Can you work these out from the model? Positions are in its coordinate system, mm. Coordinates: 2 decimals unless noted, no trailing zeros. Order: outer loops, then holes, each group sorted by start corner. A loop starts at its lowest first (then second) coordinate and runs counter-clockwise, first axis right, second up. Notation, with made-up numbers: (26, 39) -> (85, 39) arc R19 cw to (85, 71) -> close; hole circle Ø4 at (60.5, 72.25). An arc over 180 degrees is marked (long way). Answer as a JSON object with one key per item and string values. Group by question number.
(1) If we mould it in two halves opening along X, with no side actions, what happens to faces 1 (the cylindrical face through (30.228, 5.76, -0.522)), 2 (the flat face through (-4, 0, -18)), 3 (the flat face through (2, 0, 2)), 4 (the cylindrical face through (-0.522, 5.76, -30.228))? For each: pulls with the +X half, pulls with the -X half, needs draft (parallel to the pull), parting line crosses it, or undercut.
(2) For pin 1 (3 mm diameter, centred on x = 14, y = -0.5, fed in from +Z); pin 2 (5 mm diameter, centred on y = 0, z = -17, fed in from -X); pin 3 (1.5 mm diameter, centred on y = -0.5, z = 14.5, fed in from +X); pin 4 (12 mm diameter, centred on x = 19.5, z = 12, fed in from -Y), each with a flat end and sliding along its axis, tell me the tip position at first contact or that it passes through.
(3) I want a section at A-A, the plane y = 1.75. List the corners of the cut face in (x, z) for me.
(4) I want a section at C-C, the plane x = -14. List the corners of the cut face in (y, z) for me, plus the area to 3 significant figures.
(5) I need wall thicknesses on line 1 (X direction, y = 10, z = -3); line 2 (X direction, y = 5, z = -1); line 3 (Z direction, x = -16, y = -1). Which ranges of each line are inside material? Lowest first, please.
(6) I want a section at B-B, the plane y = 5.75. List the corners of the cut face in (x, z) for me.
from build123d import *

# Parameters (mm, degrees)
BOSS_EXTRU_1_DEPTH           = 3
BOSS_EXTRU_1_DEPTH_BACK      = 3
BOSS_EXTRU_2_START           = -6
ESQUISSE2_R                  = 4.01172956
BOSS_EXTRU_2_DEPTH           = 14.5
R_P_TITION_CIRCULAIRE1_COUNT = 4
ESQUISSE3_R                  = 1.05
ENL_V_MAT_EXTRU_1_DEPTH      = 43.796548364
ENL_V_MAT_EXTRU_1_DEPTH_BACK = 43.796548364
ENL_V_MAT_EXTRU_2_DEPTH      = 12.5
ENL_V_MAT_EXTRU_2_DEPTH_BACK = 4.0000001


with BuildPart() as part:
    # Esquisse1 → Boss.-Extru.1 (new body, two sides)
    with BuildSketch(Plane(origin=(0, 0, 0), x_dir=(1, 0, 0), z_dir=(0, 1, 0))) as boss_extru_1_sk:
        with BuildLine():
            Line((4, -25.943448113), (4, -9.16515139))
            ThreePointArc((4, -9.16515139), (7.071067812, -7.071067812), (9.16515139, -4))
            Line((9.16515139, -4), (25.943448113, -4))
            ThreePointArc((25.943448113, -4), (26.25, 0), (25.943448113, 4))
            Line((25.943448113, 4), (9.16515139, 4))
            ThreePointArc((9.16515139, 4), (7.071067812, 7.071067812), (4, 9.16515139))
            Line((4, 9.16515139), (4, 25.943448113))
            ThreePointArc((4, 25.943448113), (0, 26.25), (-4, 25.943448113))
            Line((-4, 25.943448113), (-4, 9.16515139))
            ThreePointArc((-4, 9.16515139), (-7.071067812, 7.071067812), (-9.16515139, 4))
            Line((-9.16515139, 4), (-25.943448113, 4))
            ThreePointArc((-25.943448113, 4), (-26.25, 0), (-25.943448113, -4))
            Line((-25.943448113, -4), (-9.16515139, -4))
            ThreePointArc((-9.16515139, -4), (-7.071067812, -7.071067812), (-4, -9.16515139))
            Line((-4, -9.16515139), (-4, -25.943448113))
            ThreePointArc((-4, -25.943448113), (0, -26.25), (4, -25.943448113))
        make_face()
    extrude(amount=BOSS_EXTRU_1_DEPTH)
    extrude(boss_extru_1_sk.sketch, amount=-BOSS_EXTRU_1_DEPTH_BACK)

    # Esquisse2 → Boss.-Extru.2 (add)
    with BuildSketch(Plane(origin=(0, 3, 0), x_dir=(1, 0, 0), z_dir=(0, 1, 0)).offset(BOSS_EXTRU_2_START)):
        with Locations((0, 26.25)):
            Circle(ESQUISSE2_R)
    boss_extru_2 = extrude(amount=BOSS_EXTRU_2_DEPTH)

    # Répétition circulaire1: Boss.-Extru.2 ×4 about axis
    r_p_tition_circulaire1_axis = Axis((0, 0, 0), (0, 1, 0))
    for i in range(1, R_P_TITION_CIRCULAIRE1_COUNT):
        add(boss_extru_2.rotate(r_p_tition_circulaire1_axis, i * 360 / R_P_TITION_CIRCULAIRE1_COUNT))

    # Esquisse3 → Enlèv. mat.-Extru.1 (cut, two sides)
    with BuildSketch(Plane(origin=(0, 0, 0), x_dir=(-0.707106781, 0, -0.707106781), z_dir=(0.707106781, 0, -0.707106781))) as enl_v_mat_extru_1_sk:
        Circle(ESQUISSE3_R)
    extrude(amount=ENL_V_MAT_EXTRU_1_DEPTH, mode=Mode.SUBTRACT)
    extrude(enl_v_mat_extru_1_sk.sketch, amount=-ENL_V_MAT_EXTRU_1_DEPTH_BACK, mode=Mode.SUBTRACT)

    # Esquisse4 → Enlèv. mat.-Extru.2 (cut, two sides)
    with BuildSketch(Plane(origin=(0, 0, 0), x_dir=(1, 0, 0), z_dir=(0, 1, 0))) as enl_v_mat_extru_2_sk:
        Polygon((-4.000103061, 0), (0, 4.000103061), (4.000103061, 0), (0, -4.000103061), align=None)
    extrude(amount=ENL_V_MAT_EXTRU_2_DEPTH, mode=Mode.SUBTRACT)
    extrude(enl_v_mat_extru_2_sk.sketch, amount=-ENL_V_MAT_EXTRU_2_DEPTH_BACK, mode=Mode.SUBTRACT)


solid = part.part
Computed values:
{
 "1": {"face 1": "undercut", "face 2": "pulls with the -X half", "face 3": "undercut", "face 4": "parting line crosses it"},
 "2": {"pin 1": "stops at z = 4", "pin 2": "stops at x = -4", "pin 3": "stops at x = 4", "pin 4": "passes through"},
 "3": {"outline": "(-25.94, -4) -> (-9.17, -4) arc R10 ccw to (-4, -9.17) -> (-4, -25.94) arc R4.01 ccw (long way) to (4, -25.94) -> (4, -9.17) arc R10 ccw to (9.17, -4) -> (25.94, -4) arc R4.01 ccw (long way) to (25.94, 4) -> (9.17, 4) arc R10 ccw to (4, 9.17) -> (4, 25.94) arc R4.01 ccw (long way) to (-4, 25.94) -> (-4, 9.17) arc R10 ccw to (-9.17, 4) -> (-25.94, 4) arc R4.01 ccw (long way) to start; hole (-4, 0) -> (0, -4) -> (4, 0) -> (0, 4) -> close"},
 "4": {"outline": "(-3, -4) -> (3, -4) -> (3, 4) -> (-3, 4) -> close", "area": "48.0 mm2"},
 "5": {"line 1": "x = -28.91 to -23.59, 23.59 to 28.91", "line 2": "x = -30.14 to -22.36, 22.36 to 30.14", "line 3": "z = -4 to 4"},
 "6": {"outline": "circle Ø8.02 at (-26.25, 0); circle Ø8.02 at (0, -26.25); circle Ø8.02 at (0, 26.25); circle Ø8.02 at (26.25, 0)"}
}
